Part print with two shaded views. Sizes in mm from the minimum x, y, z corner. A direction names the side the tool comes from. Round coordinates to 2 decimals unless told otherwise and drop trailing zeros. Write each loop counter-clockwise with the first axis right and the second up, starting at its lowest first coordinate (ties: lowest second). Pieces come first, ordered by that corner, then holes. Notation, with made-up numbers: (-29.5, 17.25) - (23.5, 17.25) arc R16 ccw to (23.5, 37.25) - close; hole circle Ø9 at (67.5, 13). An arc over 180 degrees is marked (long way). Use one line per item in the form item = value. Start each with the question number.
Item 1: Band-saw the part on B-B, the plane z = 1. List the corners of the cut face in (x, y).
Item 2: Drill centre lines: L1, parallel to X at y = 21.98, z = 0.8; L2, parallel to X at y = 21.98, z = 2.95; L3, parallel to Z at x = 37, y = 8.5. Where is each one in solid material? Low to high.
Item 3: Band-saw the part on C-C, the plane z = 6.25. List the corners of the cut face in (x, y), and give its area (3 significant figures).
Item 4: Tool access for the marked faces 4 and 5: list every direction of +Z, -Z, +X, -X, +Y, -Y with a clear straight run to the whole face (end or side of a thin tool).
Item 5: Band-saw the part on A-A, the plane y = 21.98. List the corners of the cut face in (x, z).
Item 6: Pin check, flat tips, straight feed: pin 1 (3.5 mm diameter, centred on x = 9.48, y = 21.98, fed in from +Z); pin 2 (1.5 mm diameter, centred on y = 12.5, z = 8, fed in from +X); pin 3 (1 mm diameter, centred on y = 31, z = 6, fed in from -X). Stop position of each tip, or through.
Item 7: Pull direction Y, two halves, no side cores. Call the marked faces 1, 2 and 3: +Y half, -Y half, draft (parallel to the pull), parting line (faces both ways), or undercut.
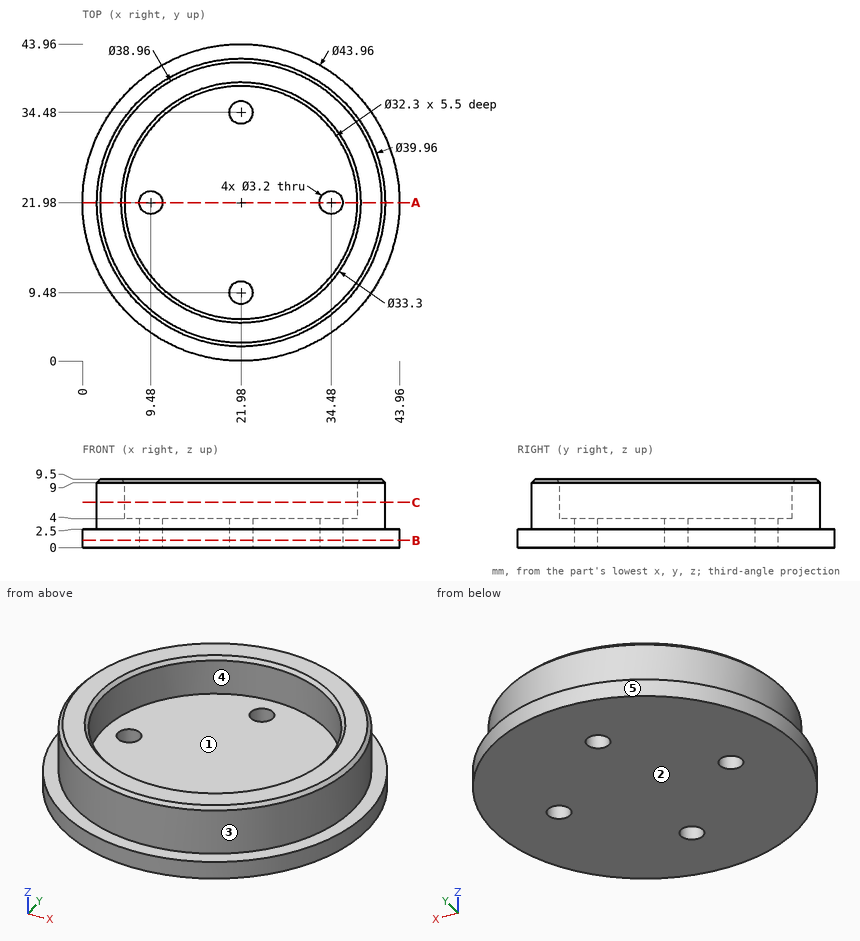
Determined:
q1.outline = circle Ø43.96 at (21.98, 21.98); hole circle Ø3.2 at (9.48, 21.98); hole circle Ø3.2 at (21.98, 9.48); hole circle Ø3.2 at (21.98, 34.48); hole circle Ø3.2 at (34.48, 21.98)
q2.L1 = 0 to 7.88, 11.08 to 32.88, 36.08 to 43.96
q2.L2 = 2 to 7.88, 11.08 to 32.88, 36.08 to 41.96
q2.L3 = 0 to 2.5
q3.outline = circle Ø39.96 at (21.98, 21.98); hole circle Ø32.3 at (21.98, 21.98)
q3.area = 435 mm²
q4.face_4 = +Z
q4.face_5 = +Z, -Z
q5.outline = (0, 0) - (7.88, 0) - (7.88, 4) - (5.83, 4) - (5.83, 9) - (5.33, 9.5) - (2.5, 9.5) - (2, 9) - (2, 2.5) - (0, 2.5) - close; (11.08, 0) - (32.88, 0) - (32.88, 4) - (11.08, 4) - close; (36.08, 0) - (43.96, 0) - (43.96, 2.5) - (41.96, 2.5) - (41.96, 9) - (41.46, 9.5) - (38.63, 9.5) - (38.13, 9) - (38.13, 4) - (36.08, 4) - close
q6.pin_1 = 4
q6.pin_2 = 39.95
q6.pin_3 = 3.91
q7.face_1 = undercut
q7.face_2 = draft
q7.face_3 = parting line
